Work out the finished part from the listing and answer in its coordinate system (mm). A direction names the side the tool comes from. Give positions to 0.01 mm unless a question says otherwise; leave off trailing zeros. Loops run counter-clockwise (first coordinate to the right, second up) from the corner with the lowest first, then second, coordinate; pieces in that order, holes last. Notation, with made-up numbers: M -5,77 L 44,77 A32 cw 44,110 Z; hole C 20.25,17 d5. An arc over 180 degrees is marked long. Answer as a JSON object with one key per item and string values. Group by question number.
```python
from build123d import *

# Parameters (mm, degrees)
SKETCH1_W           = 45
SKETCH1_H           = 45
BOSS_EXTRUDE1_DEPTH = 14
CUT_EXTRUDE1_DEPTH  = 35.763486592
CHAMFER1_SIZE       = 0.5
CHAMFER2_SIZE       = 2
SKETCH4_R           = 1.75
CUT_EXTRUDE2_DEPTH  = 35.763486592
SKETCH5_R           = 1.75
SKETCH5_W           = 4
SKETCH5_H           = 25.5
BOSS_EXTRUDE4_DEPTH = 5
SKETCH5_3_R         = 1.75
SKETCH5_3_W         = 4
SKETCH5_3_H         = 25.5
BOSS_EXTRUDE5_DEPTH = 10
SKETCH10_W          = 21
SKETCH10_H          = 6
CUT_EXTRUDE3_DEPTH  = 50
CHAMFER5_SIZE       = 0.5


with BuildPart() as part:
    # Sketch1 → Boss-Extrude1 (new body)
    with BuildSketch(Plane(origin=(0, 0, 0), x_dir=(1, 0, 0), z_dir=(0, 1, 0))):
        Rectangle(SKETCH1_W, SKETCH1_H)
    extrude(amount=BOSS_EXTRUDE1_DEPTH)

    # Sketch3 → Cut-Extrude1 (cut, through all)
    with BuildSketch(Plane(origin=(0, 14, 0), x_dir=(1, 0, 0), z_dir=(0, 1, 0))):
        with BuildLine():
            Line((-22.5, 12.75), (-8.05, 12.75))
            ThreePointArc((-8.05, 12.75), (-6.211522369, 13.511522369), (-5.45, 15.35))
            Line((-5.45, 15.35), (-5.45, 16.35))
            ThreePointArc((-5.45, 16.35), (-4.688477631, 18.188477631), (-2.85, 18.95))
            Line((-2.85, 18.95), (2.65, 18.95))
            ThreePointArc((2.65, 18.95), (4.488477631, 18.188477631), (5.25, 16.35))
            Line((5.25, 16.35), (5.25, 15.35))
            ThreePointArc((5.25, 15.35), (6.011522369, 13.511522369), (7.85, 12.75))
            Line((7.85, 12.75), (16.5, 12.75))
            Line((16.5, 12.75), (16.5, -12.75))
            Line((16.5, -12.75), (7.85, -12.75))
            ThreePointArc((7.85, -12.75), (6.011522369, -13.511522369), (5.25, -15.35))
            Line((5.25, -15.35), (5.25, -16.35))
            ThreePointArc((5.25, -16.35), (4.488477631, -18.188477631), (2.65, -18.95))
            Line((2.65, -18.95), (-2.85, -18.95))
            ThreePointArc((-2.85, -18.95), (-4.688477631, -18.188477631), (-5.45, -16.35))
            Line((-5.45, -16.35), (-5.45, -15.35))
            ThreePointArc((-5.45, -15.35), (-6.211522369, -13.511522369), (-8.05, -12.75))
            Line((-8.05, -12.75), (-22.5, -12.75))
            Line((-22.5, -12.75), (-22.5, 12.75))
        make_face()
    extrude(amount=-CUT_EXTRUDE1_DEPTH, mode=Mode.SUBTRACT)

    # Chamfer1
    chamfer1_edges = [part.edges().sort_by_distance(p)[0] for p in [
        (-22.5, 14, -17.625),
        (0, 14, 22.5),
        (-22.5, 14, 17.625),
        (22.5, 14, 0),
        (0, 14, -22.5),
    ]]
    chamfer(chamfer1_edges, length=CHAMFER1_SIZE)

    # Chamfer2
    # the kernel refuses this chamfer: 5.464101615, 2 mm, written as the material it takes off along each edge
    # the kernel refuses this chamfer: 5.464101615, 2 mm, written as the material it takes off along each edge
    with BuildSketch(Plane(origin=(-22.5, -5.143365976, -22.5), x_dir=(-0.027495876610585647, 0, 0.9996219169112968), z_dir=(0, 1, 0)), Plane(origin=(-22.5, -5.143365976, 22.5), x_dir=(0.9996219169112968, 0, 0.027495876610585647), z_dir=(0, 1, 0))) as chamfer2_2_piece_1:
        Polygon((CHAMFER2_SIZE * 0.999621916911, CHAMFER2_SIZE * 0.0274958766106), (-CHAMFER2_SIZE * 0.0274958766106, CHAMFER2_SIZE * 0.999621916911), (0, 0), align=None)
    extrude(amount=23.786731952, mode=Mode.SUBTRACT)
    with BuildSketch(Plane(origin=(22.5, -5.143365976, 22.5), x_dir=(-0.9996219169112968, 0, 0.027495876610585647), z_dir=(0, 1, 0)), Plane(origin=(22.5, -5.143365976, -22.5), x_dir=(0.027495876610585647, 0, 0.9996219169112968), z_dir=(0, 1, 0))) as chamfer2_2_piece_2:
        Polygon((CHAMFER2_SIZE * 0.999621916911, -CHAMFER2_SIZE * 0.0274958766106), (-CHAMFER2_SIZE * 0.0274958766106, -CHAMFER2_SIZE * 0.999621916911), (0, 0), align=None)
    extrude(amount=23.786731952, mode=Mode.SUBTRACT)

    # Sketch4 → Cut-Extrude2 (cut, through all)
    with BuildSketch(Plane(origin=(0, 14, 0), x_dir=(1, 0, 0), z_dir=(0, 1, 0))):
        with Locations(Location((-18, 17.25, 0), (0, 0, 270))):
            Circle(SKETCH4_R)
        with Locations(Location((18, 17.25, 0), (0, 0, 270))):
            Circle(SKETCH4_R)
        with Locations(Location((18, -17.25, 0), (0, 0, 270))):
            Circle(SKETCH4_R)
        with Locations(Location((-18, -17.25, 0), (0, 0, 270))):
            Circle(SKETCH4_R)
    extrude(amount=-CUT_EXTRUDE2_DEPTH, mode=Mode.SUBTRACT)

    # Sketch5 → Boss-Extrude4 (add)
    # profile 1 of 13: a face of its own
    with BuildSketch(Plane.XZ):
        Polygon((-20.5, 22.5), (-37.5, 22.5), (-37.5, -22.5), (-20.5, -22.5), (-22.5, -20.5), (-22.5, -12.75), (-12.5, -12.75), (-12.5, 12.75), (-22.5, 12.75), (-22.5, 20.5), align=None)
    # profile 2 of 13: a face of its own
    with BuildSketch(Plane.XZ):
        with BuildLine():
            Line((-8.05, 12.75), (-12.5, 12.75))
            Line((-12.5, 12.75), (-12.5, -12.75))
            Line((-12.5, -12.75), (-8.05, -12.75))
            ThreePointArc((-8.05, -12.75), (-6.211522369, -13.511522369), (-5.45, -15.35))
            Line((-5.45, -15.35), (-5.45, -16.35))
            ThreePointArc((-5.45, -16.35), (-4.688477631, -18.188477631), (-2.85, -18.95))
            Line((-2.85, -18.95), (2.65, -18.95))
            ThreePointArc((2.65, -18.95), (4.488477631, -18.188477631), (5.25, -16.35))
            Line((5.25, -16.35), (5.25, -15.35))
            ThreePointArc((5.25, -15.35), (6.011522369, -13.511522369), (7.85, -12.75))
            Line((7.85, -12.75), (12.5, -12.75))
            Line((12.5, -12.75), (12.5, 12.75))
            Line((12.5, 12.75), (7.85, 12.75))
            ThreePointArc((7.85, 12.75), (6.011522369, 13.511522369), (5.25, 15.35))
            Line((5.25, 15.35), (5.25, 16.35))
            ThreePointArc((5.25, 16.35), (4.488477631, 18.188477631), (2.65, 18.95))
            Line((2.65, 18.95), (-2.85, 18.95))
            ThreePointArc((-2.85, 18.95), (-4.688477631, 18.188477631), (-5.45, 16.35))
            Line((-5.45, 16.35), (-5.45, 15.35))
            ThreePointArc((-5.45, 15.35), (-6.211522369, 13.511522369), (-8.05, 12.75))
        make_face()
    # profile 3 of 13: a face of its own
    with BuildSketch(Plane.XZ):
        with BuildLine():
            Line((12.5, 22.5), (-12.5, 22.5))
            Line((-12.5, 22.5), (-12.5, 12.75))
            Line((-12.5, 12.75), (-8.05, 12.75))
            ThreePointArc((-8.05, 12.75), (-6.211522369, 13.511522369), (-5.45, 15.35))
            Line((-5.45, 15.35), (-5.45, 16.35))
            ThreePointArc((-5.45, 16.35), (-4.688477631, 18.188477631), (-2.85, 18.95))
            Line((-2.85, 18.95), (2.65, 18.95))
            ThreePointArc((2.65, 18.95), (4.488477631, 18.188477631), (5.25, 16.35))
            Line((5.25, 16.35), (5.25, 15.35))
            ThreePointArc((5.25, 15.35), (6.011522369, 13.511522369), (7.85, 12.75))
            Line((7.85, 12.75), (12.5, 12.75))
            Line((12.5, 12.75), (12.5, 22.5))
        make_face()
    # profile 4 of 13: a face of its own
    with BuildSketch(Plane.XZ):
        Polygon((-12.5, 22.5), (-20.5, 22.5), (-22.5, 20.5), (-22.5, 12.75), (-12.5, 12.75), align=None)
        with Locations(Location((-18, 17.25, 0), (0, 0, 90))):
            Circle(SKETCH5_R, mode=Mode.SUBTRACT)
    # profile 5 of 13: a face of its own
    with BuildSketch(Plane.XZ):
        Polygon((20.5, 22.5), (12.5, 22.5), (12.5, 12.75), (16.5, 12.75), (16.5, -12.75), (12.5, -12.75), (12.5, -22.5), (20.5, -22.5), (22.5, -20.5), (22.5, 20.5), align=None)
        with Locations(Location((18, -17.25, 0), (0, 0, 90))):
            Circle(SKETCH5_R, mode=Mode.SUBTRACT)
        with Locations(Location((18, 17.25, 0), (0, 0, 90))):
            Circle(SKETCH5_R, mode=Mode.SUBTRACT)
    # profile 6 of 13: a face of its own
    with BuildSketch(Plane.XZ):
        Polygon((37.5, 22.5), (20.5, 22.5), (22.5, 20.5), (22.5, -20.5), (20.5, -22.5), (37.5, -22.5), align=None)
    # profile 7 of 13: a face of its own
    with BuildSketch(Plane.XZ):
        with BuildLine():
            Line((-12.5, -12.75), (-12.5, -22.5))
            Line((-12.5, -22.5), (12.5, -22.5))
            Line((12.5, -22.5), (12.5, -12.75))
            Line((12.5, -12.75), (7.85, -12.75))
            ThreePointArc((7.85, -12.75), (6.011522369, -13.511522369), (5.25, -15.35))
            Line((5.25, -15.35), (5.25, -16.35))
            ThreePointArc((5.25, -16.35), (4.488477631, -18.188477631), (2.65, -18.95))
            Line((2.65, -18.95), (-2.85, -18.95))
            ThreePointArc((-2.85, -18.95), (-4.688477631, -18.188477631), (-5.45, -16.35))
            Line((-5.45, -16.35), (-5.45, -15.35))
            ThreePointArc((-5.45, -15.35), (-6.211522369, -13.511522369), (-8.05, -12.75))
            Line((-8.05, -12.75), (-12.5, -12.75))
        make_face()
    # profile 8 of 13: a face of its own
    with BuildSketch(Plane.XZ):
        Polygon((-22.5, -20.5), (-20.5, -22.5), (-12.5, -22.5), (-12.5, -12.75), (-22.5, -12.75), align=None)
        with Locations(Location((-18, -17.25, 0), (0, 0, 90))):
            Circle(SKETCH5_R, mode=Mode.SUBTRACT)
    # profile 9 of 13: a face of its own
    with BuildSketch(Plane.XZ):
        with Locations((14.5, 0)):
            Rectangle(SKETCH5_W, SKETCH5_H)
    # profile 10 of 13: a face of its own
    with BuildSketch(Plane.XZ):
        with Locations(Location((18, 17.25, 0), (0, 0, 90))):
            Circle(SKETCH5_R)
    # profile 11 of 13: a face of its own
    with BuildSketch(Plane.XZ):
        with Locations(Location((-18, 17.25, 0), (0, 0, 90))):
            Circle(SKETCH5_R)
    # profile 12 of 13: a face of its own
    with BuildSketch(Plane.XZ):
        with Locations(Location((-18, -17.25, 0), (0, 0, 90))):
            Circle(SKETCH5_R)
    # profile 13 of 13: a face of its own
    with BuildSketch(Plane.XZ):
        with Locations(Location((18, -17.25, 0), (0, 0, 90))):
            Circle(SKETCH5_R)
    extrude(amount=BOSS_EXTRUDE4_DEPTH)

    # Sketch5<3> → Boss-Extrude5 (add)
    # profile 1 of 10: a face of its own
    with BuildSketch(Plane.XZ):
        Polygon((-12.5, 22.5), (-20.5, 22.5), (-22.5, 20.5), (-22.5, 12.75), (-12.5, 12.75), align=None)
        with Locations(Location((-18, 17.25, 0), (0, 0, 90))):
            Circle(SKETCH5_3_R, mode=Mode.SUBTRACT)
    # profile 2 of 10: a face of its own
    with BuildSketch(Plane.XZ):
        Polygon((-20.5, 22.5), (-37.5, 22.5), (-37.5, -22.5), (-20.5, -22.5), (-22.5, -20.5), (-22.5, -12.75), (-12.5, -12.75), (-12.5, 12.75), (-22.5, 12.75), (-22.5, 20.5), align=None)
    # profile 3 of 10: a face of its own
    with BuildSketch(Plane.XZ):
        Polygon((-22.5, -20.5), (-20.5, -22.5), (-12.5, -22.5), (-12.5, -12.75), (-22.5, -12.75), align=None)
        with Locations(Location((-18, -17.25, 0), (0, 0, 90))):
            Circle(SKETCH5_3_R, mode=Mode.SUBTRACT)
    # profile 4 of 10: a face of its own
    with BuildSketch(Plane.XZ):
        with Locations(Location((-18, 17.25, 0), (0, 0, 90))):
            Circle(SKETCH5_3_R)
    # profile 5 of 10: a face of its own
    with BuildSketch(Plane.XZ):
        with Locations(Location((-18, -17.25, 0), (0, 0, 90))):
            Circle(SKETCH5_3_R)
    # profile 6 of 10: a face of its own
    with BuildSketch(Plane.XZ):
        Polygon((20.5, 22.5), (12.5, 22.5), (12.5, 12.75), (16.5, 12.75), (16.5, -12.75), (12.5, -12.75), (12.5, -22.5), (20.5, -22.5), (22.5, -20.5), (22.5, 20.5), align=None)
        with Locations(Location((18, -17.25, 0), (0, 0, 90))):
            Circle(SKETCH5_3_R, mode=Mode.SUBTRACT)
        with Locations(Location((18, 17.25, 0), (0, 0, 90))):
            Circle(SKETCH5_3_R, mode=Mode.SUBTRACT)
    # profile 7 of 10: a face of its own
    with BuildSketch(Plane.XZ):
        Polygon((37.5, 22.5), (20.5, 22.5), (22.5, 20.5), (22.5, -20.5), (20.5, -22.5), (37.5, -22.5), align=None)
    # profile 8 of 10: a face of its own
    with BuildSketch(Plane.XZ):
        with Locations((14.5, 0)):
            Rectangle(SKETCH5_3_W, SKETCH5_3_H)
    # profile 9 of 10: a face of its own
    with BuildSketch(Plane.XZ):
        with Locations(Location((18, 17.25, 0), (0, 0, 90))):
            Circle(SKETCH5_3_R)
    # profile 10 of 10: a face of its own
    with BuildSketch(Plane.XZ):
        with Locations(Location((18, -17.25, 0), (0, 0, 90))):
            Circle(SKETCH5_3_R)
    extrude(amount=BOSS_EXTRUDE5_DEPTH)

    # Sketch10 → Cut-Extrude3 (cut)
    with BuildSketch(Plane(origin=(0, 0, -22.5), x_dir=(-1, 0, 0), z_dir=(0, 0, -1))):
        with Locations((-25, -5)):
            Rectangle(SKETCH10_W, SKETCH10_H)
        with Locations((25, -5)):
            Rectangle(SKETCH10_W, SKETCH10_H)
    extrude(amount=-CUT_EXTRUDE3_DEPTH, mode=Mode.SUBTRACT)

    # Chamfer5
    chamfer5_edges = [part.edges().sort_by_distance(p)[0] for p in [
        (37.5, 0, 0),
        (-37.5, -5, -22.5),
        (37.5, -5, -22.5),
        (37.5, -5, 22.5),
        (-37.5, 0, 0),
        (-37.5, -5, 22.5),
        (-12.5, -10, 0),
        (-37.5, -10, 0),
        (37.5, -10, 0),
        (12.5, -10, 0),
    ]]
    chamfer(chamfer5_edges, length=CHAMFER5_SIZE)


solid = part.part
```
Item 1: Given pin 1 Ø8.5 at (y, z) = (9.5, -17) entering from -X; pin 2 Ø5 at (x, z) = (30.5, -5.5) entering from +Y; pin 3 Ø3 at (y, z) = (10.5, -7.5) entering from +X, each flat-ended and moving along its own axis, determine where each tip first touches the part or whether it passes through.
Item 2: A tool of negligible diameter and unlimited length cuts with its end or side. For faces 5 (the cylindrical face through (-16.265, 7.098, 17.022)), 6 (the flat face through (-25, -2, 0)), 7 (the flat face through (12.5, -7, 0)), 8 (the flat face through (-22.5, 7, -17)), 9 (the flat face through (22, 7, -21)), from which of +Z, -Z, +X, -X, +Y, -Y can it reach the whole face along a straight path? Write none if from no direction.
Item 3: A cutting plane is placed at D-D (z = -10.5). Determine the outline of the cut face in (x, y), and give its area (3 significant figures).
Item 4: A cutting plane is placed at A-A (x = 31.5). Determine the outline of the cut face in (y, z).
Item 5: Find the intervals of material crossed by probe 1 along X at (y, z) = (-7.5, -3); probe 2 along X at (y, z) = (-3.5, -12); probe 3 along Y at (x, z) = (-24.5, -5.5), in increasing order. Write a range as [from, to].
Item 6: A cutting plane is placed at B-B (y = 1). Give the number of separate pieces and of enclosed holes in the cut face, and give its area (3 significant figures).
Item 7: For a pull along Z with two mould halves and no side action, classify faces 1 (the flat face through (-12.5, -7, 0)), 2 (the cylindrical face through (-4.668, 7.098, 18.209)), 3 (the flat face through (-21, 7, 22)), 4 (the flat face through (-15, 7, -12.75)) as pulls with the +Z half, pulls with the -Z half, needs draft (parallel to the pull), parting line crosses it, or undercut.
Item 8: A cutting plane is placed at C-C (y = -4.25). Determine the outline of the cut face in (x, z), and give its area (3 significant figures).
The answers:
{
 "1": {"pin 1": "stops at x = -22.5", "pin 2": "stops at y = 0", "pin 3": "stops at x = 22.5"},
 "2": {"face 5": "+Y", "face 6": "+Z, -Z", "face 7": "+Z, -Z, -Y", "face 8": "+Z, -Z, -X, +Y", "face 9": "-Z, +X, +Y"},
 "3": {"outline": "M -37.5,-9.5 L -37,-10 L -13,-10 L -12.5,-9.5 L -12.5,-5 L 12.5,-5 L 12.5,-9.5 L 13,-10 L 37,-10 L 37.5,-9.5 L 37.5,-0.5 L 37,0 L 22.5,0 L 22.5,13.5 L 22,14 L 16.5,14 L 16.5,0 L -37,0 L -37.5,-0.5 Z; hole M -35.5,-8 L -14.5,-8 L -14.5,-2 L -35.5,-2 Z; hole M 14.5,-8 L 35.5,-8 L 35.5,-2 L 14.5,-2 Z", "area": "456 mm^2"},
 "4": {"outline": "M -10,-22.5 L -8,-22.5 L -8,22.5 L -10,22.5 Z; M -2,-22.5 L 0,-22.5 L 0,22.5 L -2,22.5 Z"},
 "5": {"probe 1": "x = [-37.5, -35.5], [-14.5, -12.5], [12.5, 14.5], [35.5, 37.5]", "probe 2": "x = [-37.5, -35.5], [-14.5, 14.5], [35.5, 37.5]", "probe 3": "y = [-10, -8], [-2, 0]"},
 "6": {"separate pieces": "1", "enclosed holes": "4", "area": "851 mm^2"},
 "7": {"face 1": "needs draft", "face 2": "undercut", "face 3": "pulls with the +Z half", "face 4": "undercut"},
 "8": {"outline": "M -37.5,-22 L -37,-22.5 L -35.5,-22.5 L -35.5,22.5 L -37,22.5 L -37.5,22 Z; M -14.5,-22.5 L 14.5,-22.5 L 14.5,22.5 L -14.5,22.5 Z; M 35.5,-22.5 L 37,-22.5 L 37.5,-22 L 37.5,22 L 37,22.5 L 35.5,22.5 Z", "area": "1,480 mm^2"}
}
